Here's how the part is built. I have some questions about the finished solid (model axes, mm). Face numbers are marked on the shaded views. A direction names the side the tool comes from. Give positions to 0.01 mm unless a question says otherwise; leave off trailing zeros. Write each loop counter-clockwise with the first axis right and the second up, starting at its lowest first coordinate (ties: lowest second). Pieces come first, ordered by that corner, then holes. Notation, with made-up numbers: (-25, 5) -> (16, 5) arc R6 ccw to (16, 15) -> close; hole circle Ø11 at (48, 56). An arc over 180 degrees is marked (long way). Use CSV: the item, a comma, the result in double quotes. Start each with the question number.
(1) For pin 1 Ø4 at (x, y) = (4.5, -2) entering from -Z; pin 2 Ø4 at (y, z) = (6, 8.5) entering from -X; pin 3 Ø1.5 at (x, z) = (0, 8.5) entering from -Y; pin 4 Ø4 at (y, z) = (6.5, 1.5) entering from +X, each with a flat end and sliding along its axis, tell me the tip position at first contact or that it passes through.
(2) If we mould it in two halves opening along Y, with no side actions, what happens to the marked faces 3, 4 and 5? For each: pulls with the +Y half, pulls with the -Y half, needs draft (parallel to the pull), parting line crosses it, or undercut.
(3) I need wall thicknesses on L1, parallel to Y at x = 0, z = 7.25; L2, parallel to X at y = 0, z = 4.75; L3, parallel to Y at x = 0, z = 2. Which ranges of each line are inside material? Lowest first, please. Write a range as [from, to].
(4) Suppose I cut it at C-C on z = 9. List the corners of the cut face in (x, y) for me (3 decimals).
(5) Suppose I cut it at D-D on x = -3.25. List the corners of the cut face in (y, z) for me.
(6) Which directions (+Z, -Z, +X, -X, +Y, -Y) give clear straight access to the entire face, cutting with the end or side of a thin tool? Please do the marked faces 1 and 2.
(7) Suppose I cut it at B-B on x = 1. List the corners of the cut face in (y, z) for me, plus the area to 3 significant figures.
(8) Suppose I cut it at A-A on y = 0. List the corners of the cut face in (x, z) for me, plus the area to 3 significant figures.
Autodesk Fusion 360 part; units mm, degrees
sketch "Sketch1" plane through (0, 0, 0) normal (0, 0, 1) x (1, 0, 0)
  circle A0 centre (0, 0) radius 10
  circle A1 centre (0, 0) radius 5.9
  circle A2 centre (0, 0) radius 2.8
  circle A3 centre (0, 0) radius 1.35
  line L0 (-0.6583, 7.8026) -> (-0.6583, 5.6186)
  arc A4 (-0.6583, 5.6186) -> (0.6417, 5.6186) centre (-0.0083, 5.6186) ccw
  line L1 (0.6417, 5.6186) -> (0.6417, 7.8026)
  arc A5 (0.6417, 7.8026) -> (-0.6583, 7.8026) centre (-0.0083, 7.8026) ccw
  line L2 (-0.0083, 7.8026) -> (-0.0083, 5.6186) construction
  dimension "d1" = 20
  dimension "d2" = 11.8
  dimension "d3" = 5.6
  dimension "d4" = 2.7
  dimension "d10" = 1.3
extrude "Extrude1" add sketch "Sketch1" along normal blind 2.8 contours A0 | A1 L0 A4 L1 | A1 L0 A4 L1 | A1 L0 L1 A5 | A2
extrude "Extrude2" add sketch "Sketch1" along normal blind 9.8 contours A1 L0 A4 L1 picked at (-1.284, 4.3991)
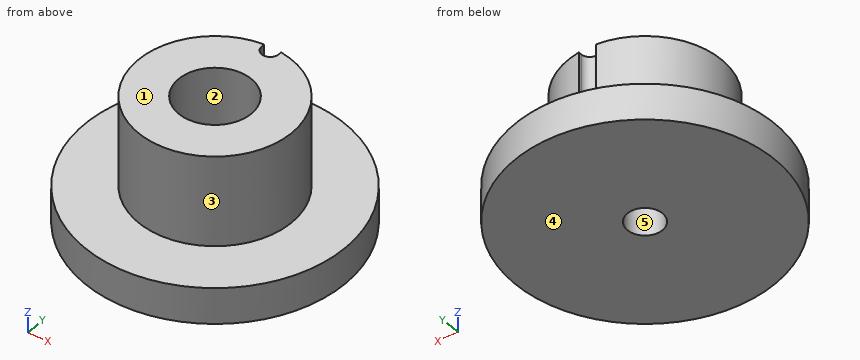
Geometry says:
1,pin 1,"z = 0"
1,pin 2,"x = -4.34"
1,pin 3,"y = -5.9"
1,pin 4,"x = 8.93"
2,face 3,"parting line crosses it"
2,face 4,"needs draft"
2,face 5,"undercut"
3,L1,"[-5.9, -2.8], [2.8, 4.97]"
3,L2,"[-5.9, -2.8], [2.8, 5.9]"
3,L3,"[-10, -1.35], [1.35, 10]"
4,outline,"(-0.658, 5.619) -> (-0.658, 5.863) arc R5.9 ccw (long way) to (0.642, 5.865) -> (0.642, 5.619) arc R0.65 cw to start; hole circle Ø5.6 at (0, 0)"
5,outline,"(-9.46, 0) -> (9.46, 0) -> (9.46, 2.8) -> (4.92, 2.8) -> (4.92, 9.8) -> (-4.92, 9.8) -> (-4.92, 2.8) -> (-9.46, 2.8) -> close"
6,face 1,"+Z, +X, -X, +Y, -Y"
6,face 2,"+Z"
7,outline,"(-9.95, 0) -> (-0.91, 0) -> (-0.91, 2.8) -> (-2.62, 2.8) -> (-2.62, 9.8) -> (-5.81, 9.8) -> (-5.81, 2.8) -> (-9.95, 2.8) -> close; (0.91, 0) -> (9.95, 0) -> (9.95, 2.8) -> (5.81, 2.8) -> (5.81, 9.8) -> (2.62, 9.8) -> (2.62, 2.8) -> (0.91, 2.8) -> close"
7,area,"95.4 mm²"
8,outline,"(-10, 0) -> (-1.35, 0) -> (-1.35, 2.8) -> (-2.8, 2.8) -> (-2.8, 9.8) -> (-5.9, 9.8) -> (-5.9, 2.8) -> (-10, 2.8) -> close; (1.35, 0) -> (10, 0) -> (10, 2.8) -> (5.9, 2.8) -> (5.9, 9.8) -> (2.8, 9.8) -> (2.8, 2.8) -> (1.35, 2.8) -> close"
8,area,"91.8 mm²"
